Geometry: see drawing. Coordinates: mm, zero at the bounding-box minimum. A direction names the side the tool comes from. Coordinates: 2 decimals unless noted, no trailing zeros. Loops run counter-clockwise (first coordinate to the right, second up) from the corner with the lowest first, then second, coordinate; pieces in that order, holes last. Notation, with made-up numbers: (33, 10.5) -> (45, 10.5) arc R19 ccw to (45, 45.5) -> close; hole circle Ø7 at (-2, 13). An arc over 180 degrees is marked (long way). Answer as a JSON object with one key per item and string values.
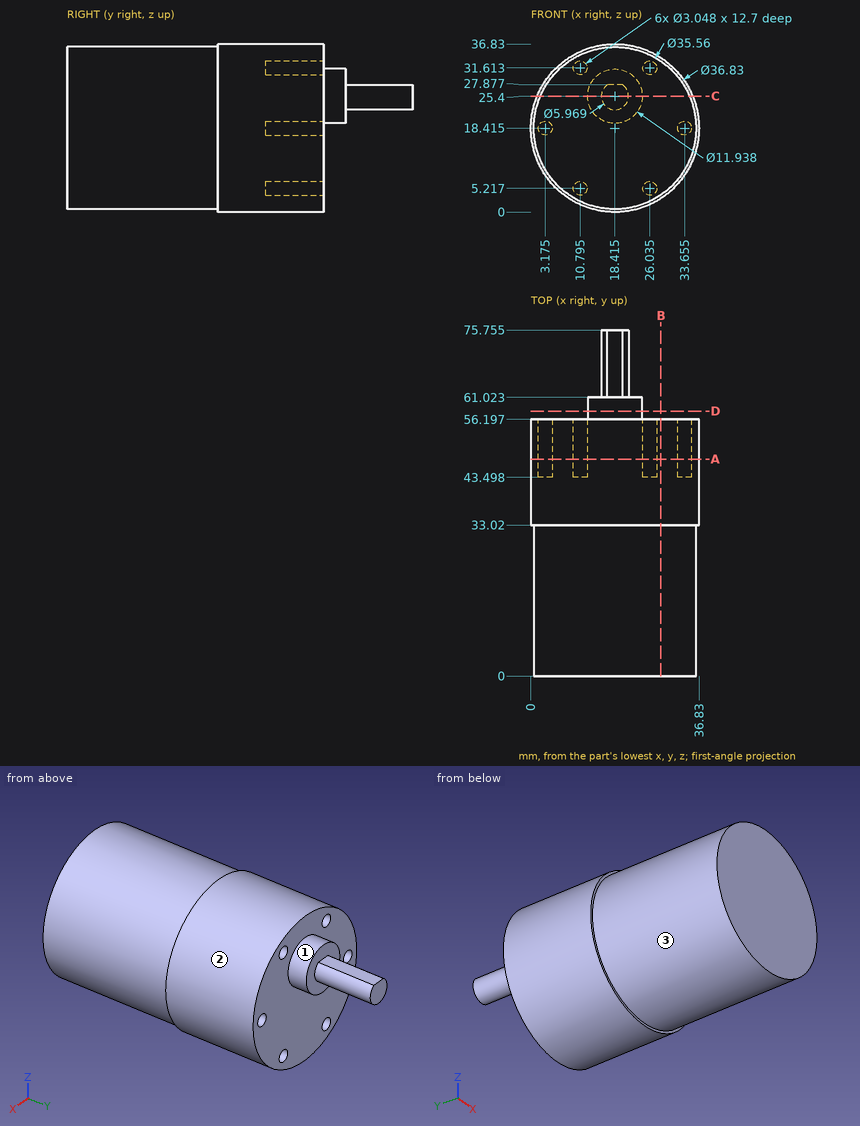
1. Section query B-B (x = 28.5). Return loops of the section in (y, z).
Reply:
{"outline": "(0, 3.77) -> (33.02, 3.77) -> (33.02, 3.01) -> (56.2, 3.01) -> (56.2, 33.82) -> (33.02, 33.82) -> (33.02, 33.06) -> (0, 33.06) -> close"}
2. Section query D-D (y = 58). Return loops of the section in (x, z) (1 decimal), plus the area to 3 significant figures.
Reply:
{"outline": "circle Ø11.9 at (18.4, 25.4)", "area": "112 mm2"}
3. Pin query (flat end, axial travel): P1, Ø2, axis at y = 52, z = 4, coming from the +X side; P2, Ø3.5, axis at x = 3.5, z = 19, coming from the +Y side; P3, Ø2.5, axis at x = 26.04, z = 31.61, coming from the +Y side. Return the tip coordinate at first contact, or that it passes through.
Reply:
{"P1": "stops at x = 31.03", "P2": "stops at y = 56.2", "P3": "stops at y = 43.5"}
4. Access query for the marked faces 1, 2 and 3. Directions: +Z, -Z, +X, -X, +Y, -Y. A direction counts if a zero-diameter tool reaches every point of the face in a straight line with its end or side. Return the directions, or none.
Reply:
{"face 1": "+Y", "face 2": "+Y, -Y", "face 3": "-Y"}
5. Section query C-C (z = 25.4). Return loops of the section in (x, y) (1 decimal), plus the area to 4 significant figures.
Reply:
{"outline": "(1.4, 33) -> (2.1, 33) -> (2.1, 0) -> (34.8, 0) -> (34.8, 33) -> (35.5, 33) -> (35.5, 56.2) -> (24.4, 56.2) -> (24.4, 61) -> (21.4, 61) -> (21.4, 75.8) -> (15.4, 75.8) -> (15.4, 61) -> (12.4, 61) -> (12.4, 56.2) -> (1.4, 56.2) -> close", "area": "2,015 mm2"}
6. Line query: line 1 along Y through (x, z) = (11.5, 23.5); line 2 along Y through (x, z) = (33.5, 17.5); line 3 along X through (y, z) = (67, 26.5). Output: solid intervals per line, ascending.
Reply:
{"line 1": "y = 0 to 56.2", "line 2": "y = 0 to 43.5", "line 3": "x = 15.64 to 21.19"}
7. Section query A-A (y = 47.5). Return loops of the section in (x, z) (1 decimal), plus the area to 3 significant figures.
Reply:
{"outline": "circle Ø36.8 at (18.4, 18.4); hole circle Ø3 at (3.2, 18.4); hole circle Ø3 at (10.8, 5.2); hole circle Ø3 at (10.8, 31.6); hole circle Ø3 at (26, 5.2); hole circle Ø3 at (26, 31.6); hole circle Ø3 at (33.7, 18.4)", "area": "1,020 mm2"}
